```python
from build123d import *

# Parameters (mm, degrees)
BOSS_EXTRUDE1_DEPTH = 10
CUT_EXTRUDE2_DEPTH  = 330
SKETCH4_W           = 178
SKETCH4_H           = 12
CUT_EXTRUDE3_DEPTH  = 2730.484566727
SKETCH5_W           = 12
SKETCH5_H           = 309
CUT_EXTRUDE4_DEPTH  = 10


with BuildPart() as part:
    # Sketch1 → Boss-Extrude1 (new body)
    with BuildSketch(Plane.XY):
        Polygon((1230, 1510), (0, 1510), (0, 0), (1685, 0), (1685, -309), (2035, -309), (2035, 1819), (1230, 1819), align=None)
    extrude(amount=BOSS_EXTRUDE1_DEPTH)

    # Sketch3 → Cut-Extrude2 (cut)
    with BuildSketch(Plane(origin=(-124.112118138, -342, 1004.457487155), x_dir=(-1, 0, 0), z_dir=(0, -1, 0))):
        with BuildLine():
            Line((-1887.112118138, 819.457487155), (-1466.112118138, 819.457487155))
            ThreePointArc((-1466.112118138, 819.457487155), (-1395.40144002, 848.746809036), (-1366.112118138, 919.457487155))
            Line((-1366.112118138, 919.457487155), (-1366.112118138, 2569.457487155))
            ThreePointArc((-1366.112118138, 2569.457487155), (-1395.40144002, 2640.168165273), (-1466.112118138, 2669.457487155))
            Line((-1466.112118138, 2669.457487155), (-1887.112118138, 2669.457487155))
            ThreePointArc((-1887.112118138, 2669.457487155), (-1957.822796257, 2640.168165273), (-1987.112118138, 2569.457487155))
            Line((-1987.112118138, 2569.457487155), (-1987.112118138, 919.457487155))
            ThreePointArc((-1987.112118138, 919.457487155), (-1957.822796257, 848.746809036), (-1887.112118138, 819.457487155))
        make_face()
    extrude(amount=-CUT_EXTRUDE2_DEPTH, mode=Mode.SUBTRACT)

    # Sketch4 → Cut-Extrude3 (cut, through all)
    with BuildSketch(Plane(origin=(0, 0, 0), x_dir=(-1, 0, 0), z_dir=(0, 0, -1))):
        with Locations((-1774, -6)):
            Rectangle(SKETCH4_W, SKETCH4_H)
    extrude(amount=-CUT_EXTRUDE3_DEPTH, mode=Mode.SUBTRACT)

    # Sketch5 → Cut-Extrude4 (cut)
    with BuildSketch(Plane(origin=(0, 0, 0), x_dir=(-1, 0, 0), z_dir=(0, 0, -1))):
        with Locations((-1869, -154.5)):
            Rectangle(SKETCH5_W, SKETCH5_H)
    extrude(amount=-CUT_EXTRUDE4_DEPTH, mode=Mode.SUBTRACT)


solid = part.part
```
The listing builds one solid part. Answer for the finished solid, in the listing's coordinates (mm). Give positions to 0.01 mm unless a question says otherwise; leave off trailing zeros. Loops run counter-clockwise (first coordinate to the right, second up) from the corner with the lowest first, then second, coordinate; pieces in that order, holes last. Notation, with made-up numbers: (17, 48.25) - (28, 48.25) arc R17 ccw to (28, 58.25) - close; hole circle Ø4 at (-19, -9). An arc over 180 degrees is marked (long way). Return JSON: item names as keys, results as strings. Group by question number.
1. Find section C-C (x = 1619). Write down the section's boundary in (y, z), then the cut area to 3 significant figures.
2. Straight lines are drawn through the part: line 1 (Y direction, x = 729.5, z = 1.25); line 2 (Y direction, x = 1258, z = 5.5); line 3 (X direction, y = 1647, z = 2.25). For each, find the intervals that lie inside material, in ascending order. Write a range as [from, to].
3. Given pin 1 Ø12 at (x, y) = (1211.5, 260) entering from -Z; pin 2 Ø1.5 at (x, z) = (1777, 3) entering from -Y; pin 3 Ø2 at (x, z) = (574, 3) entering from +Y; pin 4 Ø5 at (y, z) = (-209.5, 6) entering from -X, each flat-ended and moving along its own axis, determine where each tip first touches the part or whether it passes through.
4. Find section B-B (x = 390.5). Write down the section's boundary in (y, z), then the cut area to 3 significant figures.
5. Find section A-A (z = 5). Write down the section's boundary in (x, y), then the cut area to 3 significant figures.
Verdict:
{
 "1": {"outline": "(0, 0) - (1819, 0) - (1819, 10) - (0, 10) - close", "area": "18,200 mm^2"},
 "2": {"line 1": "y = [0, 1510]", "line 2": "y = [0, 1819]", "line 3": "x = [1230, 2035]"},
 "3": {"pin 1": "stops at z = 0", "pin 2": "stops at y = 0", "pin 3": "stops at y = 1510", "pin 4": "stops at x = 1875"},
 "4": {"outline": "(0, 0) - (1510, 0) - (1510, 10) - (0, 10) - close", "area": "15,100 mm^2"},
 "5": {"outline": "(0, 0) - (1875, 0) - (1875, -309) - (2035, -309) - (2035, 1819) - (1230, 1819) - (1230, 1510) - (0, 1510) - close", "area": "3,370,000 mm^2"}
}
